Part model, mm, in its own coordinate system. Give positions to 0.01 mm unless a question says otherwise; leave off trailing zeros. Write each loop counter-clockwise with the first axis right and the second up, starting at its lowest first coordinate (ties: lowest second). Pieces come first, ordered by that corner, then holes. Notation, with made-up numbers: (86.5, 47) - (109.5, 47) arc R22 ccw to (109.5, 58) - close; hole circle Ø3 at (-25.75, -36). An arc over 180 degrees is marked (long way). Answer in a Markdown table with one row per item. Add a question column.
1. Probe line 1 along Z through (x, y) = (1155.7, -3.5) (3 decimals); line 2 along Y through (x, z) = (664.5, 3.5). List the from-to ranges inside material, lowest first.
2. Band-saw the part on B-B on z = 14. Write the cut outline in (x, y), plus the area to 3 significant figures.
3. Band-saw the part on A-A on x = 674. Write the cut outline in (y, z).
4. Drop flat-ended pins along their axis: pin 1 Ø8.5 at (x, z) = (12.7, 6.35) entering from +Y; pin 2 Ø2 at (x, y) = (824.5, 10) entering from +Z. Give the stop position or say it passes through.
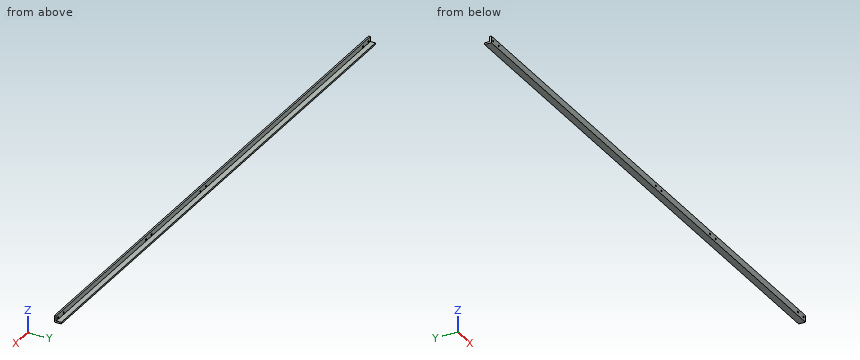
```python
from build123d import *

# Parameters (mm, degrees)
BOSS_EXTRUDE1_DEPTH = 2133.6
SKETCH2_R           = 3.175
CUT_EXTRUDE1_DEPTH  = 914.4


with BuildPart() as part:
    # Sketch1 → Boss-Extrude1 (new body)
    with BuildSketch(Plane(origin=(0, 0, 0), x_dir=(0, 0, -1), z_dir=(1, 0, 0))):
        Polygon((0, 0), (0, 19.05), (6.35, 19.05), (6.35, -6.35), (-19.05, -6.35), (-19.05, 0), align=None)
    extrude(amount=BOSS_EXTRUDE1_DEPTH)

    # Sketch2 → Cut-Extrude1 (cut)
    with BuildSketch(Plane.XZ.offset(6.35)):
        with Locations(Location((12.7, 6.35, 0), (0, 0, 270))):
            Circle(SKETCH2_R)
        with Locations(Location((50.8, 6.35, 0), (0, 0, 270))):
            Circle(SKETCH2_R)
        with Locations(Location((1117.6, 6.35, 0), (0, 0, 270))):
            Circle(SKETCH2_R)
        with Locations(Location((1155.7, 6.35, 0), (0, 0, 270))):
            Circle(SKETCH2_R)
        with Locations(Location((1485.9, 6.35, 0), (0, 0, 270))):
            Circle(SKETCH2_R)
        with Locations(Location((1524, 6.35, 0), (0, 0, 270))):
            Circle(SKETCH2_R)
        with Locations(Location((2082.8, 6.35, 0), (0, 0, 270))):
            Circle(SKETCH2_R)
        with Locations(Location((2120.9, 6.35, 0), (0, 0, 270))):
            Circle(SKETCH2_R)
    extrude(amount=-CUT_EXTRUDE1_DEPTH, mode=Mode.SUBTRACT)


solid = part.part
```
Values:
| question | item | result |
|---|---|---|
| 1 | line 1 | z = -6.35 to 3.175, 9.525 to 19.05 |
| 1 | line 2 | y = -6.35 to 0 |
| 2 | outline | (0, -6.35) - (2133.6, -6.35) - (2133.6, 0) - (0, 0) - close |
| 2 | area | 13,500 mm² |
| 3 | outline | (-6.35, -6.35) - (19.05, -6.35) - (19.05, 0) - (0, 0) - (0, 19.05) - (-6.35, 19.05) - close |
| 4 | pin 1 | stops at y = 0 |
| 4 | pin 2 | stops at z = 0 |
